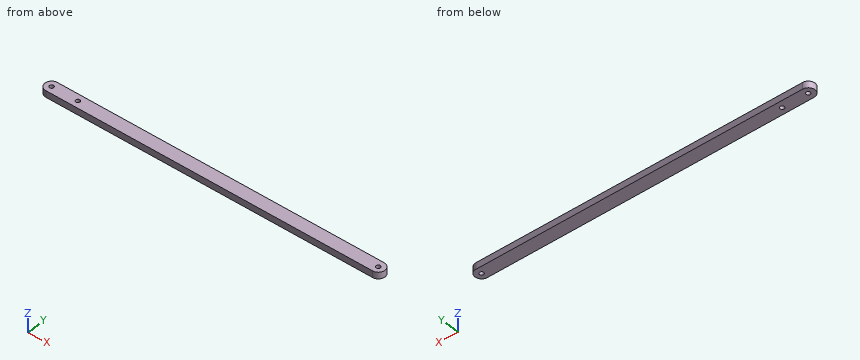
from build123d import *

# Parameters (mm, degrees)
SKETCH1_R           = 2.032
BOSS_EXTRUDE1_DEPTH = 3.175


with BuildPart() as part:
    # Sketch1 → Boss-Extrude1 (new, symmetric)
    with BuildSketch(Plane.XY):
        with BuildLine():
            Line((0, 6.35), (317.5, 6.35))
            ThreePointArc((317.5, 6.35), (323.85, 0), (317.5, -6.35))
            Line((317.5, -6.35), (0, -6.35))
            ThreePointArc((0, -6.35), (-6.35, 0), (0, 6.35))
        make_face()
        Circle(SKETCH1_R, mode=Mode.SUBTRACT)
        with Locations((317.5, 0)):
            Circle(SKETCH1_R, mode=Mode.SUBTRACT)
        with Locations((25.4, 0)):
            Circle(SKETCH1_R, mode=Mode.SUBTRACT)
    extrude(amount=BOSS_EXTRUDE1_DEPTH, both=True)


solid = part.part
Source: CAD feature listing. Evaluate the final solid. Frame: model axes, mm. Round coordinates to 2 decimals unless told otherwise and drop trailing zeros. Order: outer loops, then holes, each group sorted by start corner. A loop starts at its lowest first (then second) coordinate and runs counter-clockwise, first axis right, second up. Notation, with made-up numbers: (85, -30.5) -> (97, -30.5) arc R33 cw to (97, 1.5) -> close; hole circle Ø11 at (19.25, 11.25). An arc over 180 degrees is marked (long way). Answer as CSV lines item,"result".
Item 1: Section B-B, the plane z = 1.5. Return loops of the section in (x, y), plus the area to 3 significant figures.
A:
outline,"(0, -6.35) -> (317.5, -6.35) arc R6.35 ccw to (317.5, 6.35) -> (0, 6.35) arc R6.35 ccw to start; hole circle Ø4.06 at (0, 0); hole circle Ø4.06 at (25.4, 0); hole circle Ø4.06 at (317.5, 0)"
area,"4,120 mm²"
Item 2: Section A-A, the plane y = 0. Return loops of the section in (x, z) (3 decimals), plus the area to 3 significant figures.
A:
outline,"(-6.35, -3.175) -> (-2.032, -3.175) -> (-2.032, 3.175) -> (-6.35, 3.175) -> close; (2.032, -3.175) -> (23.368, -3.175) -> (23.368, 3.175) -> (2.032, 3.175) -> close; (27.432, -3.175) -> (315.468, -3.175) -> (315.468, 3.175) -> (27.432, 3.175) -> close; (319.532, -3.175) -> (323.85, -3.175) -> (323.85, 3.175) -> (319.532, 3.175) -> close"
area,"2,020 mm²"
Item 3: Line query: L1, parallel to Y at x = 25.4, z = 0.25; L2, parallel to X at y = -2.25, z = -1; L3, parallel to X at y = 3.25, z = -2. Output: solid intervals per line, ascending.
A:
L1,"-6.35 to -2.03, 2.03 to 6.35"
L2,"-5.94 to 323.44"
L3,"-5.46 to 322.96"
Item 4: Pin query (flat end, axial travel): pin 1 Ø5.5 at (x, y) = (0, 0) entering from -Z (3 decimals); pin 2 Ø3.5 at (x, y) = (25.4, 0) entering from +Z; pin 3 Ø1.5 at (y, z) = (-2.5, 1) entering from +X. Return the tip coordinate at first contact, or that it passes through.
A:
pin 1,"z = -3.175"
pin 2,"through"
pin 3,"x = 323.6"
